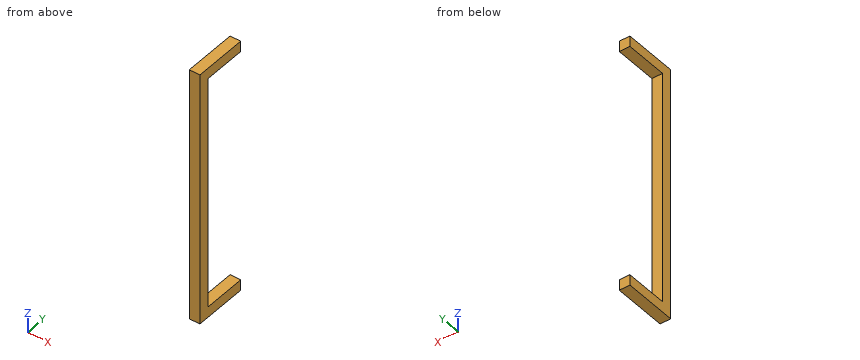
```python
from build123d import *

# Parameters (mm, degrees)
ESQUISSE1_W        = 5
ESQUISSE1_H        = 5
BOSS_EXTRU_1_DEPTH = 120.28
ESQUISSE3_W        = 5
ESQUISSE3_H        = 5
BOSS_EXTRU_2_DEPTH = 20


with BuildPart() as part:
    # Esquisse1 → Boss.-Extru.1 (new body)
    with BuildSketch(Plane.XY):
        Rectangle(ESQUISSE1_W, ESQUISSE1_H)
    extrude(amount=BOSS_EXTRU_1_DEPTH)

    # Esquisse3 → Boss.-Extru.2 (add)
    with BuildSketch(Plane(origin=(0, 2.5, 0), x_dir=(1, 0, 0), z_dir=(0, 1, 0))):
        with Locations((0, -2.5)):
            Rectangle(ESQUISSE3_W, ESQUISSE3_H)
        with Locations((0, -117.78)):
            Rectangle(ESQUISSE3_W, ESQUISSE3_H)
    extrude(amount=BOSS_EXTRU_2_DEPTH)


solid = part.part
```
Geometry: final body of the model. Coordinates: model frame, mm. Coordinates: 2 decimals unless noted, no trailing zeros. Order: outer loops, then holes, each group sorted by start corner. A loop starts at its lowest first (then second) coordinate and runs counter-clockwise, first axis right, second up. Notation, with made-up numbers: M -0.5,39 L 18.5,39 A17 cw 18.5,64 Z; hole C 20,-1 d3. An arc over 180 degrees is marked long. Answer in a Markdown table with one row per item. Add a question column.
Q1. Section query B-B on x = 0.35. Return the cut outline in (y, z), and give its area (3 significant figures).
Q2. Line query: L1, parallel to Z at x = 2, y = 9; L2, parallel to Y at x = 2, z = 90.5. Output: solid intervals per line, ascending.
Q3. Contact query for a flat-ended pin moving along its axis: P1, Ø2.5, axis at x = 1, z = 71.5, coming from the +Y side. Output: stop coordinate, or through.
Q4. Section query A-A on y = 4.5. Return the cut outline in (x, z), and give its area (3 significant figures).
Q5. Section query C-C on z = 53. Return the cut outline in (x, y).
Completed:
| question | item | result |
|---|---|---|
| 1 | outline | M -2.5,0 L 22.5,0 L 22.5,5 L 2.5,5 L 2.5,115.28 L 22.5,115.28 L 22.5,120.28 L -2.5,120.28 Z |
| 1 | area | 801 mm2 |
| 2 | L1 | z = 0 to 5, 115.28 to 120.28 |
| 2 | L2 | y = -2.5 to 2.5 |
| 3 | P1 | stops at y = 2.5 |
| 4 | outline | M -2.5,0 L 2.5,0 L 2.5,5 L -2.5,5 Z; M -2.5,115.28 L 2.5,115.28 L 2.5,120.28 L -2.5,120.28 Z |
| 4 | area | 50.0 mm2 |
| 5 | outline | M -2.5,-2.5 L 2.5,-2.5 L 2.5,2.5 L -2.5,2.5 Z |
